The listing builds one solid part. Answer for the finished solid, in the listing's coordinates (mm). Round coordinates to 2 decimals unless told otherwise and drop trailing zeros. Write each loop counter-clockwise with the first axis right and the second up, starting at its lowest first coordinate (ties: lowest second). Pieces come first, ordered by that corner, then holes. Notation, with made-up numbers: (-21, 1.25) - (-7, 1.25) arc R29 ccw to (-7, 33.25) - close; hole circle Ø2 at (-5, 24). An arc over 180 degrees is marked (long way). Use a Markdown table: item, result. Add a question column.
1) A cutting plane is placed at B-B (z = 2.1). State how many separate pieces and enclosed holes the cut face has, then the cut area to 3 significant figures.
2) A cutting plane is placed at A-A (x = 136). Give the vertices of the cut face in (y, z).
3) A cutting plane is placed at C-C (x = 127.5). Give the vertices of the cut face in (y, z), then the cut area to 3 significant figures.
4) Each of these flat-tipped pins is pushed along its axis until it touches: P1, Ø1.5, axis at x = 96, z = 2, coming from the -Y side; P2, Ø1, axis at y = -97.5, z = 1, coming from the +X side. Where does it stop, or does it pass through?
5) A cutting plane is placed at D-D (y = -99.5). Give the vertices of the cut face in (x, z).
6) Find the intervals of material crossed by probe 1 along Y at (x, z) = (105.5, 1.6); probe 2 along Y at (x, z) = (86, 2.55); probe 3 along X at (y, z) = (-123, 2.55), in increasing order. Write a range as from..to.
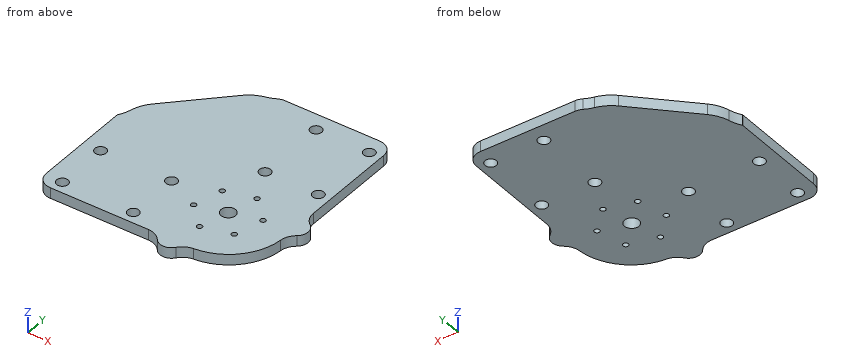
```python
from build123d import *

# Parameters (mm, degrees)
SKETCH1_R           = 0.75
SKETCH1_R_2         = 2.05
SKETCH1_R_3         = 1.6
BOSS_EXTRUDE1_DEPTH = 3
CUT_EXTRUDE2_DEPTH  = 3
FILLET1_START       = -1
FILLET1_DEPTH       = 5
FILLET1_2_DEPTH     = 3


with BuildPart() as part:
    # Sketch1 → Boss-Extrude1 (new body)
    with BuildSketch(Plane.XY):
        with BuildLine():
            Line((76.776362435, -141.065631197), (112.004342533, -141.065631197))
            ThreePointArc((112.004342533, -141.065631197), (114.223405945, -141.585033293), (115.981434881, -143.035328167))
            ThreePointArc((115.981434881, -143.035328167), (118.582167111, -144.31559365), (121.170471257, -143.010385054))
            ThreePointArc((121.170471257, -143.010385054), (122.762010679, -141.623937155), (124.783836945, -141.017757268))
            ThreePointArc((124.783836945, -141.017757268), (134.526700016, -136.525786306), (139.018670978, -126.782923235))
            ThreePointArc((139.018670978, -126.782923235), (139.624850866, -124.761096969), (141.011298764, -123.169557547))
            ThreePointArc((141.011298764, -123.169557547), (142.31650736, -120.5812534), (141.036241877, -117.980521171))
            ThreePointArc((141.036241877, -117.980521171), (139.585947004, -116.222492234), (139.066544907, -114.003428823))
            Line((139.066544907, -114.003428823), (139.066544907, -78.7754981))
            ThreePointArc((139.066544907, -78.7754981), (141.336583349, -75.865660283), (139.066544907, -72.955822465))
            ThreePointArc((139.066544907, -72.955822465), (136.675727861, -69.984491924), (133.029767481, -68.865660283))
            Line((133.029767481, -68.865660283), (117.643399217, -68.865660283))
            ThreePointArc((117.643399217, -68.865660283), (113.997438837, -69.984491924), (111.60662179, -72.955822465))
            ThreePointArc((111.60662179, -72.955822465), (109.382649666, -75.341946816), (110.650765895, -78.347196))
            add(Edge.make_bspline(
                [(110.650765895, -78.347196), (109.91906925, -79.898232812), (107.925256124, -82.271997183), (105.135443821, -83.525315829), (103.882990325, -83.818107321)],
                knots=[-0.902991905, -0.902991905, -0.902991905, -0.902991905, -0.38699657, 0, 0, 0, 0], degree=3, weights=[1, 1, 1, 1, 1]))
            add(Edge.make_bspline(
                [(103.882990325, -83.818107321), (102.079131121, -84.239803321), (100.398199973, -85.1745908), (99.088288993, -86.484502541)],
                knots=[0, 0, 0, 0, 0.557222971, 0.557222971, 0.557222971, 0.557222971], degree=3, weights=[1, 1, 1, 1]))
            Line((99.088288993, -86.484502541), (84.485352307, -101.08744771))
            add(Edge.make_bspline(
                [(84.485352307, -101.08744771), (83.175441742, -102.397359036), (82.240655409, -104.078290075), (81.818960273, -105.882148879)],
                knots=[0.344558041, 0.344558041, 0.344558041, 0.344558041, 0.901042549, 0.901042549, 0.901042549, 0.901042549], degree=3, weights=[1, 1, 1, 1]))
            add(Edge.make_bspline(
                [(81.818960273, -105.882148879), (81.428573164, -107.552083308), (79.976526739, -110.290981661), (77.511343468, -112.101144248), (76.34806998, -112.649918673)],
                knots=[0.442078245, 0.442078245, 0.442078245, 0.442078245, 0.957761165, 1.344523278, 1.344523278, 1.344523278, 1.344523278], degree=3, weights=[1, 1, 1, 1, 1]))
            ThreePointArc((76.34806998, -112.649918673), (73.342799133, -111.381774562), (70.956667683, -113.605784292))
            ThreePointArc((70.956667683, -113.605784292), (67.985343813, -115.996601782), (66.866515059, -119.642557902))
            Line((66.866515059, -119.642557902), (66.866515059, -135.028857587))
            ThreePointArc((66.866515059, -135.028857587), (67.985343813, -138.674813706), (70.956667683, -141.065631197))
            ThreePointArc((70.956667683, -141.065631197), (73.866515059, -143.335707744), (76.776362435, -141.065631197))
        make_face()
        with Locations((129.079908052, -131.091021895)):
            Circle(SKETCH1_R, mode=Mode.SUBTRACT)
        with Locations((120.86953867, -133.290983741)):
            Circle(SKETCH1_R, mode=Mode.SUBTRACT)
        with Locations((114.861843981, -127.277234232)):
            Circle(SKETCH1_R, mode=Mode.SUBTRACT)
        with Locations((117.059092978, -119.070206821)):
            Circle(SKETCH1_R, mode=Mode.SUBTRACT)
        with Locations((125.27217521, -116.866903003)):
            Circle(SKETCH1_R, mode=Mode.SUBTRACT)
        with Locations((123.069502622, -125.080616499)):
            Circle(SKETCH1_R_2, mode=Mode.SUBTRACT)
        with Locations((131.279869898, -122.880652512)):
            Circle(SKETCH1_R, mode=Mode.SUBTRACT)
        with Locations((85.366524977, -122.715631197)):
            Circle(SKETCH1_R_3, mode=Mode.SUBTRACT)
        with Locations((85.366524977, -137.715631197)):
            Circle(SKETCH1_R_3, mode=Mode.SUBTRACT)
        with Locations((105.366524977, -137.715631197)):
            Circle(SKETCH1_R_3, mode=Mode.SUBTRACT)
        with Locations((105.366524977, -122.715631197)):
            Circle(SKETCH1_R_3, mode=Mode.SUBTRACT)
        with Locations((135.716544907, -87.365719383)):
            Circle(SKETCH1_R_3, mode=Mode.SUBTRACT)
        with Locations((120.716544907, -87.365719383)):
            Circle(SKETCH1_R_3, mode=Mode.SUBTRACT)
        with Locations((120.716544907, -107.365719383)):
            Circle(SKETCH1_R_3, mode=Mode.SUBTRACT)
        with Locations((135.716544907, -107.365719383)):
            Circle(SKETCH1_R_3, mode=Mode.SUBTRACT)
    extrude(amount=BOSS_EXTRUDE1_DEPTH)

    # Sketch2 → Cut-Extrude2 (cut)
    with BuildSketch(Plane(origin=(0, 0, 0), x_dir=(-1, 0, 0), z_dir=(0, 0, -1))):
        Polygon((-139.066544907, -82.365719383), (-107.206390326, -82.365719383), (-105.489345494, -66.543961021), (-134.526700016, -61.302844114), (-151.077173689, -66.543961021), align=None)
        Polygon((-64.544828407, -107.48854343), (-80.366589508, -109.20556302), (-80.366640336, -141.065717602), (-64.544901135, -153.076371625), (-59.303757824, -136.525906313), align=None)
    extrude(amount=-CUT_EXTRUDE2_DEPTH, mode=Mode.SUBTRACT)

    # Fillet1: read off the stored shape, not the designer's step
    # Fillet1 outline → Fillet1 (cut)
    with BuildSketch(Plane.XY.offset(FILLET1_START)):
        with BuildLine():
            Line((80.366640336, -141.065631197), (84.366633955, -141.065631197))
            ThreePointArc((84.366633955, -141.065631197), (81.538209086, -139.894060578), (80.366633955, -137.065637579))
            Line((80.366633955, -137.065637579), (80.366640336, -141.065631197))
        make_face()
        with BuildLine():
            add(Edge.make_bspline(
                [(107.206390326, -82.365719383), (106.946532094, -82.541418076), (106.678265015, -82.704743583), (106.402886758, -82.855136258)],
                knots=[-0.365754194, -0.365754194, -0.365754194, -0.365754194, -0.271346383, -0.271346383, -0.271346383, -0.271346383], degree=3))
            ThreePointArc((106.402886758, -82.855136258), (107.330765678, -82.490004449), (108.320125951, -82.365719383))
            Line((108.320125951, -82.365719383), (107.206390326, -82.365719383))
        make_face()
        with BuildLine():
            Line((139.066544907, -82.365719383), (135.066544907, -82.365719383))
            ThreePointArc((135.066544907, -82.365719383), (137.894972032, -83.537292258), (139.066544907, -86.365719383))
            Line((139.066544907, -86.365719383), (139.066544907, -82.365719383))
        make_face()
    extrude(amount=FILLET1_DEPTH, mode=Mode.SUBTRACT)

    # Fillet1 2 outline → Fillet1 2 (add)
    with BuildSketch(Plane.XY):
        with BuildLine():
            ThreePointArc((80.364665709, -109.205354245), (80.366108628, -109.267368328), (80.366589705, -109.329397329))
            Line((80.366589705, -109.329397329), (80.366589508, -109.20556302))
            Line((80.366589508, -109.20556302), (80.364665709, -109.205354245))
        make_face()
    extrude(amount=FILLET1_2_DEPTH)


solid = part.part
```
Entries:
| question | item | result |
|---|---|---|
| 1 | separate pieces | 1 |
| 1 | enclosed holes | 15 |
| 1 | area | 3,060 mm² |
| 2 | outline | (-134.82, 0) - (-108.94, 0) - (-108.94, 3) - (-134.82, 3) - close; (-105.79, 0) - (-88.94, 0) - (-88.94, 3) - (-105.79, 3) - close; (-85.79, 0) - (-82.48, 0) - (-82.48, 3) - (-85.79, 3) - close |
| 3 | outline | (-140.56, 0) - (-82.37, 0) - (-82.37, 3) - (-140.56, 3) - close |
| 3 | area | 175 mm² |
| 4 | P1 | stops at y = -141.07 |
| 4 | P2 | stops at x = 139.07 |
| 5 | outline | (86.07, 0) - (139.07, 0) - (139.07, 3) - (86.07, 3) - close |
| 6 | probe 1 | y = -141.07..-139.31, -136.12..-124.31, -121.12..-83.29 |
| 6 | probe 2 | y = -141.07..-139.18, -136.25..-124.18, -121.25..-99.57 |
| 6 | probe 3 | x = 80.37..83.79, 86.94..103.79, 106.94..130.54, 132.02..141.22 |
